Read the model definition and answer for the solid it produces. Units are mm, in the model's axes. Face numbers are marked on the shaded views. A direction names the side the tool comes from. Round coordinates to 2 decimals unless told otherwise and drop trailing zeros. Order: outer loops, then holes, each group sorted by start corner. A loop starts at its lowest first (then second) coordinate and runs counter-clockwise, first axis right, second up. Notation, with made-up numbers: (4.5, -6.75) - (52.5, -6.75) arc R26 ccw to (52.5, 8.25) - close; hole circle Ø4 at (65.25, 89). An arc over 180 degrees is marked (long way). Put each result on its own line as item: value. Start each with the question number.
Q1. Section A-A on x = 0.8 is taken. Give the vertices of the cut face in (y, z) (1 decimal), then the cut area to 3 significant figures.
Q2. Find the intervals of material crossed by line 1 along Z through (x, y) = (1.2, 0) (3 decimals); line 2 along Y through (x, z) = (3.05, 0); line 3 along Y through (x, z) = (1.95, 0), in increasing order. Write a range as from..to.
Q3. Which of the six approach directions +Z, -Z, +X, -X, +Y, -Y give full straight-line access (tool end or side, diameter ignored) to the marked faces 1 and 2?
Q4. Section C-C on x = 2.85 is taken. Give the vertices of the cut face in (y, z).
Q5. Each of these flat-tipped pins is pushed along its axis until it touches: pin 1 Ø1 at (x, y) = (2.5, -3) entering from +Z; pin 2 Ø1.9 at (y, z) = (0, 0) entering from +X. Where does it stop, or does it pass through?
Q6. Section B-B on x = 1.95 is taken. Give the vertices of the cut face in (y, z) (1 decimal).
Q7. For a pull along Z with two mould halves and no side action, classify the marked faces 3, 4, 5 and 6 as pulls with the +Z half, pulls with the -Z half, needs draft (parallel to the pull), parting line crosses it, or undercut.
Autodesk Inventor part; units mm, degrees
ref_plane "Work Plane1" through (10.5464, 0, 0) normal (0, 0, 1) x (-1, 0, 0)
ref_plane "YZ Plane" through (0, 0, 0) normal (1, 0, 0) x (0, 1, 0)
ref_plane "XZ Plane" through (0, 0, 0) normal (0, 1, 0) x (-1, 0, 0)
sketch "Sketch1" plane through (0, 0, 0) normal (1, 0, 0) x (0, 1, 0)
  line L0 (-3.6662, 0) -> (-1.8331, 3.175)
  line L1 (-1.8331, 3.175) -> (1.8331, 3.175)
  line L2 (1.8331, 3.175) -> (3.6662, 0)
  line L3 (3.6662, 0) -> (1.8331, -3.175)
  line L4 (1.8331, -3.175) -> (-1.8331, -3.175)
  line L5 (-1.8331, -3.175) -> (-3.6662, 0)
  point P0 (0, 0)
  point P1 (0, 0)
  dimension "d0" = 7.3323
extrude "Body" add sketch "Sketch1" along normal blind 4.1402
sketch "Sketch2" plane through (0, 0, 0) normal (-1, 0, 0) x (0, 0, 1)
  line L0 (0, -5.1326) -> (0, 5.1326)
  line L1 (-4.445, 0) -> (4.445, 0)
  point P0 (0, 0)
hole "Thread" at (0, 0, 0) direction (1, 0, 0) diameter 2.1565 end through all
chamfer "Chamfer1" distance 0.3437 angle 30 1 edges at (0, 0, -1.0782) measured on face at (0, -2.1289, -1.2625)
chamfer "Chamfer2" distance 0.3437 angle 30 1 edges at (4.1402, 0, -1.0782) measured on face at (4.1402, -2.1289, -1.2625)
sketch "Sketch3" plane through (0, 0, 0) normal (0, 0, 1) x (1, 0, 0)
  line L0 (0, 1.8331) -> (0, 3.6662)
  line L1 (0, 3.6662) -> (4.1402, 3.6662)
  line L2 (4.1402, 1.8331) -> (4.1402, 3.6662)
  line L3 (-0.828, 0) -> (4.9682, 0)
  line L4 (0.2836, 3.6662) -> (0, 3.175)
  line L5 (4.1402, 2.6987) -> (3.352, 2.6987)
  line L6 (3.352, 2.6987) -> (1.6764, 3.6662)
  dimension "d3" = 30
  dimension "d5" = 6.35
  dimension "d6" = 5.3975
  dimension "d8" = 60
  dimension "d9" = 1.6764
revolve "Chamfer3" cut sketch "Sketch3" angle 360 about axis through (-10, 0, 0) along (1, 0, 0)
ref_plane "Work Plane1" through (10.5464, 0, 0) normal (0, 0, 1) x (-1, 0, 0)
equation "\"d0\" = 1.1547 * SW"
equation "\"d1\" = KOH"
equation "\"d3\" = ANG1"
equation "\"d5\" = SW0"
equation "\"d6\" = SW1"
equation "\"d8\" = ANG2"
equation "\"d9\" = KOH1"
equation "\"d10\" = -0.5 * GD1 + 0.5 * NND"
equation "\"d39\" = -0.5 * GD1 + 0.5 * NND"
equation "\"d12\" = -0.5 * GD1 + 0.5 * NND"
equation "\"d40\" = -0.5 * GD1 + 0.5 * NND"
equation "\"ANG1\" = 30deg"
equation "\"ANG2\" = 60deg"
equation "\"NND\" = 2.8448"
equation "\"KOH\" = 4.1402"
equation "\"SW\" = 6.35"
equation "\"SW0\" = SW"
equation "\"SW1\" = 0.85 * SW"
equation "\"KOH1\" = 1.6764"
equation "\"THREADDIA\" = 2.8448"
equation "\"TOA\" = 30deg"
equation "\"E0\" = 1.155 * SW"
properties part number "IFI 100/107 - No. 4 - 40 Metal Type" material "Steel, Mild"
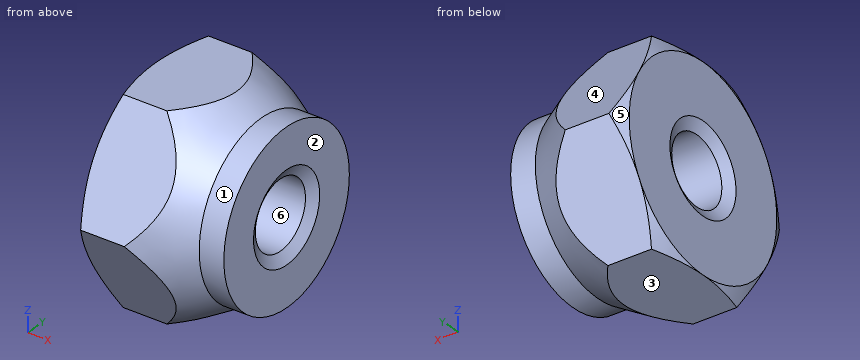
Findings:
1. outline: (-3.7, 0) - (-1.8, -3.2) - (1.8, -3.2) - (3.7, 0) - (1.8, 3.2) - (-1.8, 3.2) - close; hole circle Ø2.2 at (0, 0)
1. area: 31.3 mm2
2. line 1: -3.175..-1.078, 1.078..3.175
2. line 2: -2.87..-1.08, 1.08..2.87
2. line 3: -3.51..-1.08, 1.08..3.51
3. face 1: +X
3. face 2: +Z, -Z, +X, +Y, -Y
4. outline: circle Ø5.98 at (0, 0); hole circle Ø2.16 at (0, 0)
5. pin 1: z = 2.02
5. pin 2: through
6. outline: (-3.5, -0.3) - (-2, -2.9) arc R3.5 ccw to (-1.5, -3.2) - (1.5, -3.2) arc R3.5 ccw to (2, -2.9) - (3.5, -0.3) arc R3.5 ccw to (3.5, 0.3) - (2, 2.9) arc R3.5 ccw to (1.5, 3.2) - (-1.5, 3.2) arc R3.5 ccw to (-2, 2.9) - (-3.5, 0.3) arc R3.5 ccw to start; hole circle Ø2.2 at (0, 0)
7. face 3: pulls with the -Z half
7. face 4: pulls with the +Z half
7. face 5: parting line crosses it
7. face 6: undercut
